The model under review builds one solid part; all positions refer to its coordinate system, in mm. Round coordinates to 2 decimals unless told otherwise and drop trailing zeros. Order: outer loops, then holes, each group sorted by start corner. A loop starts at its lowest first (then second) coordinate and runs counter-clockwise, first axis right, second up.
1) Consider section A-A (y = 0.45). Give the boundary of the cut face in (x, z), then the cut area to 3 significant figures.
2) Consider section D-D (x = 14.5). Give the boundary of the cut face in (y, z).
3) Clearance check with flat-ended pins moving along their axes: P1, Ø0.8, axis at x = 12, z = -0.5, coming from the -Y side; P2, Ø5, axis at x = 23, z = 4, coming from the -Y side; P3, Ø0.8, axis at x = -0.5, y = 1.5, coming from the -Z side. State where each tip first meets the part, or that it passes through.
4) Consider section B-B (x = 32.5). Give the boundary of the cut face in (y, z).
5) To check wall thickness, follow L1, parallel to X at y = 2.6, z = 10.5; L2, parallel to Z at x = 34, y = 1.1; L3, parallel to Z at x = 33, y = 2.8. State the ranges of each line that lie inside material, in increasing order.
6) Consider section C-C (z = 2.25). Give the boundary of the cut face in (x, y).
from build123d import *

# Parameters (mm, degrees)
SKETCH_1_W          = 42
SKETCH_1_H          = 21
EXTRUDE_1_DEPTH     = 3
SKETCH_2_R          = 3
CUT_EXTRUDE_4_DEPTH = 3
CUT_EXTRUDE_6_DEPTH = 2.5
SKETCH_5_W          = 21
SKETCH_5_H          = 1
EXTRUDE_2_DEPTH     = 1
SKETCH_7_W          = 42
SKETCH_7_H          = 1
EXTRUDE_3_DEPTH     = 1
SKETCH_8_W          = 21
SKETCH_8_H          = 1
EXTRUDE_4_DEPTH     = 1


with BuildPart() as part:
    # Sketch 1 → Extrude 1 (new body)
    with BuildSketch(Plane(origin=(0, 0, 0), x_dir=(1, 0, 0), z_dir=(0, 1, 0))):
        with Locations((21, -10.5)):
            Rectangle(SKETCH_1_W, SKETCH_1_H)
    extrude(amount=EXTRUDE_1_DEPTH)

    # Sketch 2 → Cut-Extrude 4 (cut)
    with BuildSketch(Plane.XZ):
        with Locations(Location((9, 10.5, 0), (0, 0, 270))):
            Circle(SKETCH_2_R)
        with Locations(Location((17, 10.5, 0), (0, 0, 270))):
            Circle(SKETCH_2_R)
        with Locations(Location((25, 10.5, 0), (0, 0, 270))):
            Circle(SKETCH_2_R)
        with Locations(Location((33, 10.5, 0), (0, 0, 270))):
            Circle(SKETCH_2_R)
    extrude(amount=-CUT_EXTRUDE_4_DEPTH, mode=Mode.SUBTRACT)

    # Sketch 2_5 → Cut-Extrude 6 (cut)
    with BuildSketch(Plane.XZ):
        with BuildLine():
            Line((9, 13.5), (6, 13.5))
            Line((6, 13.5), (6, 10.5))
            ThreePointArc((6, 10.5), (6.878679656, 12.621320344), (9, 13.5))
        make_face()
        with BuildLine():
            ThreePointArc((9, 7.5), (6.878679656, 8.378679656), (6, 10.5))
            Line((6, 10.5), (6, 7.5))
            Line((6, 7.5), (9, 7.5))
        make_face()
        with BuildLine():
            Line((12, 13.5), (9, 13.5))
            ThreePointArc((9, 13.5), (11.121320344, 12.621320344), (12, 10.5))
            Line((12, 10.5), (12, 13.5))
        make_face()
        with BuildLine():
            Line((12, 7.5), (12, 10.5))
            ThreePointArc((12, 10.5), (11.121320344, 8.378679656), (9, 7.5))
            Line((9, 7.5), (12, 7.5))
        make_face()
        with BuildLine():
            Line((17, 13.5), (14, 13.5))
            Line((14, 13.5), (14, 10.5))
            ThreePointArc((14, 10.5), (14.878679656, 12.621320344), (17, 13.5))
        make_face()
        with BuildLine():
            ThreePointArc((17, 7.5), (14.878679656, 8.378679656), (14, 10.5))
            Line((14, 10.5), (14, 7.5))
            Line((14, 7.5), (17, 7.5))
        make_face()
        with BuildLine():
            Line((20, 13.5), (17, 13.5))
            ThreePointArc((17, 13.5), (19.121320344, 12.621320344), (20, 10.5))
            Line((20, 10.5), (20, 13.5))
        make_face()
        with BuildLine():
            Line((20, 7.5), (20, 10.5))
            ThreePointArc((20, 10.5), (19.121320344, 8.378679656), (17, 7.5))
            Line((17, 7.5), (20, 7.5))
        make_face()
        with BuildLine():
            Line((25, 13.5), (22, 13.5))
            Line((22, 13.5), (22, 10.5))
            ThreePointArc((22, 10.5), (22.878679656, 12.621320344), (25, 13.5))
        make_face()
        with BuildLine():
            Line((28, 13.5), (25, 13.5))
            ThreePointArc((25, 13.5), (27.121320344, 12.621320344), (28, 10.5))
            Line((28, 10.5), (28, 13.5))
        make_face()
        with BuildLine():
            ThreePointArc((25, 7.5), (22.878679656, 8.378679656), (22, 10.5))
            Line((22, 10.5), (22, 7.5))
            Line((22, 7.5), (25, 7.5))
        make_face()
        with BuildLine():
            Line((28, 7.5), (28, 10.5))
            ThreePointArc((28, 10.5), (27.121320344, 8.378679656), (25, 7.5))
            Line((25, 7.5), (28, 7.5))
        make_face()
        with BuildLine():
            Line((33, 13.5), (30, 13.5))
            Line((30, 13.5), (30, 10.5))
            ThreePointArc((30, 10.5), (30.878679656, 12.621320344), (33, 13.5))
        make_face()
        with BuildLine():
            ThreePointArc((33, 7.5), (30.878679656, 8.378679656), (30, 10.5))
            Line((30, 10.5), (30, 7.5))
            Line((30, 7.5), (33, 7.5))
        make_face()
        with BuildLine():
            Line((36, 13.5), (33, 13.5))
            ThreePointArc((33, 13.5), (35.121320344, 12.621320344), (36, 10.5))
            Line((36, 10.5), (36, 13.5))
        make_face()
        with BuildLine():
            Line((36, 7.5), (36, 10.5))
            ThreePointArc((36, 10.5), (35.121320344, 8.378679656), (33, 7.5))
            Line((33, 7.5), (36, 7.5))
        make_face()
    extrude(amount=-CUT_EXTRUDE_6_DEPTH, mode=Mode.SUBTRACT)

    # Sketch 5 → Extrude 2 (add)
    with BuildSketch(Plane(origin=(42, 0, 0), x_dir=(0, 0, -1), z_dir=(1, 0, 0))):
        with Locations((-10.5, 1.5)):
            Rectangle(SKETCH_5_W, SKETCH_5_H)
    extrude(amount=EXTRUDE_2_DEPTH)

    # Sketch 7 → Extrude 3 (add)
    with BuildSketch(Plane(origin=(0, 0, 0), x_dir=(-1, 0, 0), z_dir=(0, 0, -1))):
        with Locations((-21, 1.5)):
            Rectangle(SKETCH_7_W, SKETCH_7_H)
    extrude(amount=EXTRUDE_3_DEPTH)

    # Sketch 8 → Extrude 4 (add)
    with BuildSketch(Plane.ZY):
        with Locations((10.5, 1.5)):
            Rectangle(SKETCH_8_W, SKETCH_8_H)
    extrude(amount=EXTRUDE_4_DEPTH)


solid = part.part
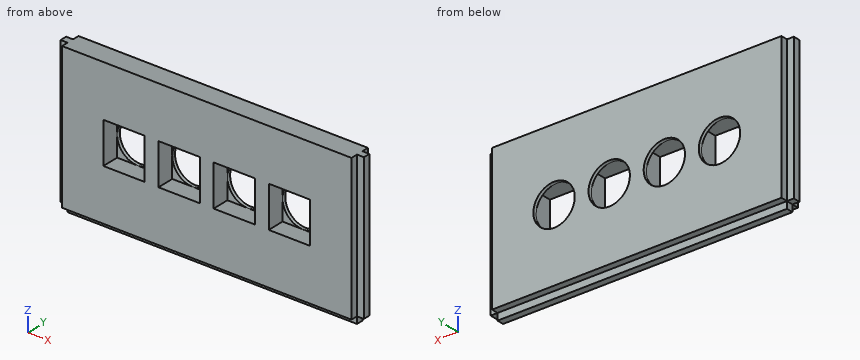
Answer below:
1. outline: (0, 0) - (42, 0) - (42, 21) - (0, 21) - close; hole (6, 7.5) - (12, 7.5) - (12, 13.5) - (6, 13.5) - close; hole (14, 7.5) - (20, 7.5) - (20, 13.5) - (14, 13.5) - close; hole (22, 7.5) - (28, 7.5) - (28, 13.5) - (22, 13.5) - close; hole (30, 7.5) - (36, 7.5) - (36, 13.5) - (30, 13.5) - close
1. area: 738 mm2
2. outline: (0, 0) - (1, 0) - (1, -1) - (2, -1) - (2, 0) - (3, 0) - (3, 8.84) - (2.5, 8.84) - (2.5, 7.5) - (0, 7.5) - close; (0, 13.5) - (2.5, 13.5) - (2.5, 12.16) - (3, 12.16) - (3, 21) - (0, 21) - close
3. P1: stops at y = 1
3. P2: stops at y = 0
3. P3: stops at z = 0
4. outline: (0, 0) - (1, 0) - (1, -1) - (2, -1) - (2, 0) - (3, 0) - (3, 7.54) - (2.5, 7.54) - (2.5, 7.5) - (0, 7.5) - close; (0, 13.5) - (2.5, 13.5) - (2.5, 13.46) - (3, 13.46) - (3, 21) - (0, 21) - close
5. L1: x = 0 to 6, 12 to 14, 20 to 22, 28 to 30, 36 to 42
5. L2: z = -1 to 7.5, 13.5 to 21
5. L3: z = 0 to 7.5, 13.5 to 21
6. outline: (-1, 1) - (0, 1) - (0, 0) - (42, 0) - (42, 1) - (43, 1) - (43, 2) - (42, 2) - (42, 3) - (0, 3) - (0, 2) - (-1, 2) - close
